Here's how the part is built. I have some questions about the finished solid (model axes, mm). Face numbers are marked on the shaded views. A direction names the side the tool comes from. Coordinates: 2 decimals unless noted, no trailing zeros. Write each loop counter-clockwise with the first axis right and the second up, starting at its lowest first coordinate (ties: lowest second). Pieces come first, ordered by that corner, then holes. Notation, with made-up numbers: (39.5, 25.5) - (82.5, 25.5) arc R14 ccw to (82.5, 46.5) - close; hole circle Ø6 at (87, 55). An arc over 180 degrees is marked (long way). Answer in a Markdown table with one row per item. Add a question column.
Item 1: If I drill on probe 1 along Z at (x, y) = (0, 0.95); probe 2 along Y at (x, z) = (11, 11), over which ranges is the centre line in solid material (lowest first)? Write a range as from..to.
Item 2: I'm going to push flat-ended pins straight in: pin 1 (2 mm diameter, centred on y = 3, z = 4, fed in from +X); pin 2 (3.5 mm diameter, centred on y = 11.5, z = 2, fed in from +X); pin 3 (2.5 mm diameter, centred on x = 4, z = 6, fed in from +Y). Where does each tip first touch, or does it pass through?
Item 3: Imagine slicing it at C-C (y = 19). Please give me the cut outline in (x, z).
Item 4: Imagine slicing it at D-D (x = -6). Please give me the cut outline in (y, z).
Item 5: Imagine slicing it at B-B (x = 0). Please give me the cut outline in (y, z).
Item 6: Which directions (+Z, -Z, +X, -X, +Y, -Y) give clear straight access to the entire face, cutting with the end or side of a thin tool? Please do the marked faces 4, 5 and 6.
Item 7: Imagine slicing it at A-A (z = 6). Please give me the cut outline in (x, y).
Item 8: We'd pull the mould along Y, two halves only. Please class the marked faces 1, 2 and 3: +Y half, -Y half, draft (parallel to the pull), parting line (faces both ways), or undercut.
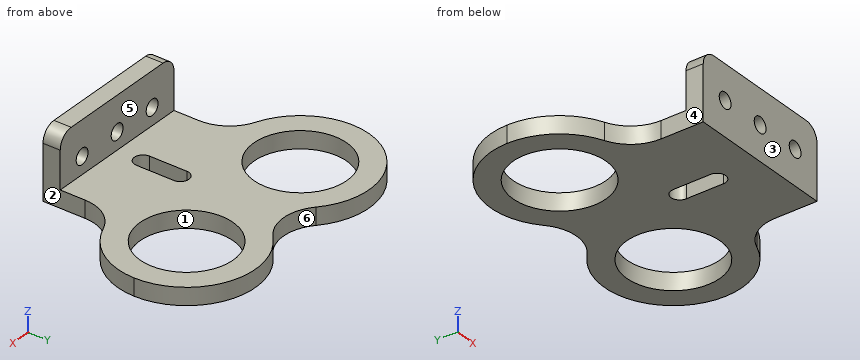
from build123d import *

# Parameters (mm, degrees)
SKETCH1_R           = 8.1
BOSS_EXTRUDE1_DEPTH = 3
SKETCH3_R           = 1.35
BOSS_EXTRUDE2_DEPTH = 3


with BuildPart() as part:
    # Sketch1 → Boss-Extrude1 (new body)
    with BuildSketch(Plane.XY):
        with BuildLine():
            Line((-13, 7.336478267), (-13, 0))
            Line((-13, 0), (13, 0))
            Line((13, 0), (13, 7.336478267))
            ThreePointArc((13, 7.336478267), (14.209808657, 11.270138676), (17.421052632, 13.844091537))
            ThreePointArc((17.421052632, 13.844091537), (22.926042302, 18.256582157), (25, 25))
            ThreePointArc((25, 25), (17.848843081, 35.976735433), (4.918546537, 33.87074461))
            ThreePointArc((4.918546537, 33.87074461), (0, 31.966212419), (-4.918546537, 33.87074461))
            ThreePointArc((-4.918546537, 33.87074461), (-17.848843081, 35.976735433), (-25, 25))
            ThreePointArc((-25, 25), (-22.926042302, 18.256582157), (-17.421052632, 13.844091537))
            ThreePointArc((-17.421052632, 13.844091537), (-14.209808657, 11.270138676), (-13, 7.336478267))
        make_face()
        with BuildLine():
            ThreePointArc((-1.5, 14), (0, 15.5), (1.5, 14))
            Line((1.5, 14), (1.5, 7.5))
            ThreePointArc((1.5, 7.5), (0, 6), (-1.5, 7.5))
            Line((-1.5, 7.5), (-1.5, 14))
        make_face(mode=Mode.SUBTRACT)
        with Locations((-13, 25)):
            Circle(SKETCH1_R, mode=Mode.SUBTRACT)
        with Locations((13, 25)):
            Circle(SKETCH1_R, mode=Mode.SUBTRACT)
    extrude(amount=BOSS_EXTRUDE1_DEPTH)

    # Sketch3 → Boss-Extrude2 (add)
    with BuildSketch(Plane.XZ):
        with BuildLine():
            Line((-13, 3), (13, 3))
            Line((13, 3), (13, 9.5))
            ThreePointArc((13, 9.5), (12.267766953, 11.267766953), (10.5, 12))
            Line((10.5, 12), (-10.5, 12))
            ThreePointArc((-10.5, 12), (-12.267766953, 11.267766953), (-13, 9.5))
            Line((-13, 9.5), (-13, 3))
        make_face()
        with Locations((8, 6)):
            Circle(SKETCH3_R, mode=Mode.SUBTRACT)
        with Locations((-8, 6)):
            Circle(SKETCH3_R, mode=Mode.SUBTRACT)
        with Locations((0, 6)):
            Circle(SKETCH3_R, mode=Mode.SUBTRACT)
    extrude(amount=-BOSS_EXTRUDE2_DEPTH)


solid = part.part
Here are the results:
| question | item | result |
|---|---|---|
| 1 | probe 1 | z = 0..4.65, 7.35..12 |
| 1 | probe 2 | y = 0..3 |
| 2 | pin 1 | stops at x = 13 |
| 2 | pin 2 | stops at x = 16.25 |
| 2 | pin 3 | stops at y = 3 |
| 3 | outline | (-23.39, 0) - (-18.44, 0) - (-18.44, 3) - (-23.39, 3) - close; (-7.56, 0) - (7.56, 0) - (7.56, 3) - (-7.56, 3) - close; (18.44, 0) - (23.39, 0) - (23.39, 3) - (18.44, 3) - close |
| 4 | outline | (0, 0) - (20.92, 0) - (20.92, 3) - (3, 3) - (3, 12) - (0, 12) - close; (29.08, 0) - (34.75, 0) - (34.75, 3) - (29.08, 3) - close |
| 5 | outline | (0, 0) - (6, 0) - (6, 3) - (3, 3) - (3, 4.65) - (0, 4.65) - close; (0, 7.35) - (3, 7.35) - (3, 12) - (0, 12) - close; (15.5, 0) - (31.97, 0) - (31.97, 3) - (15.5, 3) - close |
| 6 | face 4 | +Z, -Z, -X, -Y |
| 6 | face 5 | +Z, +X, -X, +Y |
| 6 | face 6 | +Z, -Z, +Y |
| 7 | outline | (-13, 0) - (-9.35, 0) - (-9.35, 3) - (-13, 3) - close; (-6.65, 0) - (-1.35, 0) - (-1.35, 3) - (-6.65, 3) - close; (1.35, 0) - (6.65, 0) - (6.65, 3) - (1.35, 3) - close; (9.35, 0) - (13, 0) - (13, 3) - (9.35, 3) - close |
| 8 | face 1 | undercut |
| 8 | face 2 | draft |
| 8 | face 3 | -Y half |
